The model under review builds one solid part; all positions refer to its coordinate system, in mm. A direction names the side the tool comes from. Round coordinates to 2 decimals unless told otherwise and drop trailing zeros. Loops run counter-clockwise (first coordinate to the right, second up) from the corner with the lowest first, then second, coordinate; pieces in that order, holes last. Notation, with made-up numbers: M 1.5,25.5 L 13.5,25.5 A8 ccw 13.5,40.5 Z; hole C 58,-14.5 d9. An arc over 180 degrees is marked long. Return JSON: item names as keys, results as strings. Group by question number.
Q1. Clearance check with flat-ended pins moving along their axes: pin 1 Ø1.1 at (x, z) = (-2, 0) entering from -Y; pin 2 Ø4 at (x, y) = (-2, -31) entering from -Z; pin 3 Ø4 at (x, y) = (3.5, -9.5) entering from +Z. State where each tip first meets the part, or that it passes through.
Q2. Consider section A-A (y = -16). State the section outline as (x, z) points.
Q3. Draft analysis for pull direction Z (two halves, no side actions). For faces 1 (the face through (0, -27, 0)), 2 (the face through (-1, -30, 1.143)), 3 (the face through (-1.19, 2.56, -5.37)), 4 (the face through (0, -35, -3)), state which applies: pulls with the +Z half, pulls with the -Z half, needs draft (parallel to the pull), parting line crosses it, or undercut.
Q4. To check wall thickness, follow line 1 along Z through (x, y) = (-1.5, -29); line 2 along Y through (x, z) = (0.5, -3); line 3 along Y through (x, z) = (0.25, 3.5). State the ranges of each line that lie inside material, in increasing order.
Q5. For faces 5 (the face through (-1, -30, -1.143)), 6 (the face through (-0.17, -30.11, -3.29)), 7 (the face through (4, -21.758, -3)), list the 3-axis set-ups (+Z, -Z, +X, -X, +Y, -Y) from which the entire face can be reached by the end or side of a thin tool; tool diameter is ignored.
from build123d import *

# Parameters (mm, degrees)
F0_R     = 5.5
F1_DEPTH = 35
F2_SIZE2 = 8.6602540378
F2_SIZE  = 5
F4_W     = 13.5426148772
F4_H     = 2.286007395
F5_DEPTH = 8
F6_R     = 1.3316742147
F7_DEPTH = 10
F8_W     = 1.2
F8_H     = 1.4649596699
F8_H_2   = 0.745677419


with BuildPart() as f1:
    # F0 (on Front) → F1 (new body, symmetric)
    with BuildSketch(Plane.XZ):
        Circle(F0_R)
    extrude(amount=F1_DEPTH, both=True)

    # F2
    f2_edges = [f1.edges().sort_by_distance(p)[0] for p in [
        (-5.5, 35, 0),
    ]]
    f2_side = f1.faces().sort_by_distance((0, 35, 0))[0]
    chamfer(f2_edges, length=F2_SIZE, length2=F2_SIZE2, reference=f2_side)

    # F4 (on face) → F5 (cut)
    with BuildSketch(Plane.XZ.offset(35)):
        Rectangle(F4_W, F4_H)
    extrude(amount=-F5_DEPTH, mode=Mode.SUBTRACT)

    # F6 (on Top) → F7 (cut, symmetric)
    with BuildSketch(Plane.XY):
        with Locations((0, -31.4301326871)):
            Circle(F6_R)
    extrude(amount=F7_DEPTH, both=True, mode=Mode.SUBTRACT)

    # F8 (on Right) → F9 (revolve, cut)
    with BuildSketch(Plane.YZ):
        with Locations((-21.1584017664, 6.2324798349)):
            Rectangle(F8_W, F8_H)
        with Locations((-21.1584017664, 5.1271612905)):
            Rectangle(F8_W, F8_H_2)
    revolve(axis=Axis((0, -17.5, 0), (0, 1, 0)), mode=Mode.SUBTRACT)


with BuildPart() as f10_1:
    # F10: copy of F1
    add(f1.part.moved(Location((0, 0, 34))))


with BuildPart() as f12_1:
    # F12: copy of F1
    add(f1.part)


solid = f12_1.part
Values:
{
 "1": {"pin 1": "stops at y = -27", "pin 2": "stops at z = -5.5", "pin 3": "stops at z = 5.29"},
 "2": {"outline": "C 0,0 d11"},
 "3": {"face 1": "undercut", "face 2": "undercut", "face 3": "parting line crosses it", "face 4": "needs draft"},
 "4": {"line 1": "z = -5.29 to -1.14, 1.14 to 5.29", "line 2": "y = -35 to -32.66, -30.2 to 30.6", "line 3": "y = -35 to -32.74, -30.12 to 29.79"},
 "5": {"face 5": "+X, -X, -Y", "face 6": "+Z, -Z", "face 7": "none"}
}
